from build123d import *

# Parameters (mm, degrees)
CROQUIS1_W              = 180
CROQUIS1_H              = 60
SALIENTE_EXTRUIR1_DEPTH = 3
CROQUIS2_W              = 20
CROQUIS2_H              = 3
CROQUIS2_W_2            = 13
CROQUIS2_H_2            = 20
CROQUIS2_W_3            = 7
CROQUIS2_H_3            = 14
SALIENTE_EXTRUIR2_DEPTH = 23


with BuildPart() as part:
    # Croquis1 → Saliente-Extruir1 (new body)
    with BuildSketch(Plane.XY):
        with Locations((-124.847250917, 17.903225806)):
            Rectangle(CROQUIS1_W, CROQUIS1_H)
        Polygon((-43.458800443, 44.903225806), (-123.208800443, 44.903225806), (-83.333800443, 19.678168249), align=None, mode=Mode.SUBTRACT)
        Polygon((-123.208800443, 41.353340922), (-123.208800443, -5.546889309), (-86.139575206, 17.903225806), align=None, mode=Mode.SUBTRACT)
        Polygon((-166.360701391, 19.678168249), (-126.485701391, 44.903225806), (-206.235701391, 44.903225806), align=None, mode=Mode.SUBTRACT)
        Polygon((-211.847250917, 44.903225806), (-169.166476154, 17.903225806), (-211.847250917, -9.096774194), align=None, mode=Mode.SUBTRACT)
        Polygon((-206.235701391, -9.096774194), (-166.360701391, 16.128283364), (-126.485701391, -9.096774194), align=None, mode=Mode.SUBTRACT)
        Polygon((-126.485701391, -5.546889309), (-163.554926629, 17.903225806), (-126.485701391, 41.353340922), align=None, mode=Mode.SUBTRACT)
        Polygon((-43.458800443, -9.096774194), (-83.333800443, 16.128283364), (-123.208800443, -9.096774194), align=None, mode=Mode.SUBTRACT)
        Polygon((-37.847250917, 44.903225806), (-80.52802568, 17.903225806), (-37.847250917, -9.096774194), align=None, mode=Mode.SUBTRACT)
    extrude(amount=SALIENTE_EXTRUIR1_DEPTH)

    # Croquis2 → Saliente-Extruir2 (add)
    # profile 1 of 4: a face of its own
    with BuildSketch(Plane.XY.offset(3)):
        with Locations((-204.847250917, -10.596774194)):
            Rectangle(CROQUIS2_W, CROQUIS2_H)
    # profile 2 of 4: a face of its own
    with BuildSketch(Plane.XY.offset(3)):
        with Locations((-218.347250917, 37.903225806)):
            Rectangle(CROQUIS2_W_2, CROQUIS2_H_2)
        with Locations((-218.347250917, 37.903225806)):
            Rectangle(CROQUIS2_W_3, CROQUIS2_H_3, mode=Mode.SUBTRACT)
    # profile 3 of 4: a face of its own
    with BuildSketch(Plane.XY.offset(3)):
        with Locations((-31.347250917, 37.903225806)):
            Rectangle(CROQUIS2_W_2, CROQUIS2_H_2)
        with Locations((-31.347250917, 37.903225806)):
            Rectangle(CROQUIS2_W_3, CROQUIS2_H_3, mode=Mode.SUBTRACT)
    # profile 4 of 4: a face of its own
    with BuildSketch(Plane.XY.offset(3)):
        with Locations((-44.847250917, -10.596774194)):
            Rectangle(CROQUIS2_W, CROQUIS2_H)
    extrude(amount=-SALIENTE_EXTRUIR2_DEPTH)


solid = part.part
Source: CAD feature listing. Evaluate the final solid. Frame: model axes, mm. A direction names the side the tool comes from. Give positions to 0.01 mm unless a question says otherwise; leave off trailing zeros. Loops run counter-clockwise (first coordinate to the right, second up) from the corner with the lowest first, then second, coordinate; pieces in that order, holes last. Notation, with made-up numbers: (60.5, -18.5) -> (98.5, -18.5) arc R34 ccw to (98.5, 19.5) -> close; hole circle Ø4 at (-1.5, 8). An arc over 180 degrees is marked (long way). Use a Markdown table: item, result. Add a question column.
1) Section query C-C, the plane y = 10. Return the cut outline in (x, z), then the cut area to 3 significant figures.
2) Reachability of faces 4 (the face through (-24.847, 38, -8)), 5 (the face through (-221.847, 38, -8)), 6 (the face through (-214.847, 3, 1)) from +Z, -Z, +X, -X, +Y, -Y: full face, straight path, thin tool, end or side. Return the list, or none.
3) Section query D-D, the plane y = 34. Count the separate pieces of the cut face and the enclosed holes in it, then the cut area to 3 significant figures.
4) Line query: line 1 along X through (y, z) = (-7.5, 1.25); line 2 along X through (y, z) = (28.5, -2.25); line 3 along Z through (x, y) = (-185, 29). Output: solid intervals per line, ascending. Write a range as [from, to].
5) Section query B-B, the plane x = -198.5. Return the cut outline in (y, z).
6) Pull-direction query (Y, two-part tool) for faces 1 (the face through (-125, 20, 0)), 2 (the face through (-125, -12.097, 2)), 3 (the face through (-211.847, 32, -6)); classes: +Y half, -Y half, draft (parallel to the pull), parting line (faces both ways), or undercut.
7) First-contact query: pin 1 (7 mm diameter, centred on y = 15.5, z = -4, fed in from +X); pin 2 (5.5 mm diameter, centred on x = -219, z = -9.5, fed in from -Y); pin 3 (1.5 mm diameter, centred on x = -214, y = 3.5, fed in from -Z). Flat tips, straight axial feed; report the tip coordinate or a pass-through.
8) Section query A-A, the plane z = -10.5. Return the cut outline in (x, y), then the cut area to 3 significant figures.
Numbers:
| question | item | result |
|---|---|---|
| 1 | outline | (-214.85, 0) -> (-211.85, 0) -> (-211.85, 3) -> (-214.85, 3) -> close; (-181.66, 0) -> (-176.05, 0) -> (-176.05, 3) -> (-181.66, 3) -> close; (-156.67, 0) -> (-151.06, 0) -> (-151.06, 3) -> (-156.67, 3) -> close; (-126.49, 0) -> (-123.21, 0) -> (-123.21, 3) -> (-126.49, 3) -> close; (-98.63, 0) -> (-93.02, 0) -> (-93.02, 3) -> (-98.63, 3) -> close; (-73.65, 0) -> (-68.03, 0) -> (-68.03, 3) -> (-73.65, 3) -> close; (-37.85, 0) -> (-34.85, 0) -> (-34.85, 3) -> (-37.85, 3) -> close |
| 1 | area | 95.2 mm2 |
| 2 | face 4 | +Z, -Z, +X, +Y, -Y |
| 2 | face 5 | +Z, -Z |
| 2 | face 6 | +Z, -Z, -X, -Y |
| 3 | separate pieces | 9 |
| 3 | enclosed holes | 0 |
| 3 | area | 353 mm2 |
| 4 | line 1 | x = [-214.85, -211.85], [-209.32, -203.71], [-129.01, -120.68], [-45.98, -40.37], [-37.85, -34.85] |
| 4 | line 2 | x = [-224.85, -211.85], [-37.85, -24.85] |
| 4 | line 3 | z = [0, 3] |
| 5 | outline | (-12.1, -20) -> (-9.1, -20) -> (-9.1, 3) -> (-12.1, 3) -> close; (-4.2, 0) -> (-0.65, 0) -> (-0.65, 3) -> (-4.2, 3) -> close; (36.46, 0) -> (40.01, 0) -> (40.01, 3) -> (36.46, 3) -> close; (44.9, 0) -> (47.9, 0) -> (47.9, 3) -> (44.9, 3) -> close |
| 6 | face 1 | draft |
| 6 | face 2 | -Y half |
| 6 | face 3 | undercut |
| 7 | pin 1 | passes through |
| 7 | pin 2 | stops at y = 27.9 |
| 7 | pin 3 | stops at z = 0 |
| 8 | outline | (-224.85, 27.9) -> (-211.85, 27.9) -> (-211.85, 47.9) -> (-224.85, 47.9) -> close; (-214.85, -12.1) -> (-194.85, -12.1) -> (-194.85, -9.1) -> (-214.85, -9.1) -> close; (-54.85, -12.1) -> (-34.85, -12.1) -> (-34.85, -9.1) -> (-54.85, -9.1) -> close; (-37.85, 27.9) -> (-24.85, 27.9) -> (-24.85, 47.9) -> (-37.85, 47.9) -> close; hole (-221.85, 30.9) -> (-214.85, 30.9) -> (-214.85, 44.9) -> (-221.85, 44.9) -> close; hole (-34.85, 30.9) -> (-27.85, 30.9) -> (-27.85, 44.9) -> (-34.85, 44.9) -> close |
| 8 | area | 444 mm2 |
